Work out the finished part from the listing and answer in its coordinate system (mm). A direction names the side the tool comes from. Coordinates: 2 decimals unless noted, no trailing zeros. Order: outer loops, then holes, each group sorted by start corner. A loop starts at its lowest first (then second) coordinate and runs counter-clockwise, first axis right, second up. Notation, with made-up numbers: M 60,-7.5 L 107,-7.5 A7 cw 107,3.5 Z; hole C 60.5,68 d5. An arc over 180 degrees is marked long. Use a Markdown table: item, result.
from build123d import *

# Parameters (mm, degrees)
F0_W     = 8.736010408
F0_H     = 2.1122291218
F0_H_2   = 1.7872701865
F0_W_2   = 2.455455251
F0_H_3   = 5.8963275515
F0_W_3   = 2.8000103775
F1_DEPTH = 50
F2_DEPTH = 15
F2_TAPER = -41.9


with BuildPart() as f1:
    # F0 (on Right) → F1 (new body)
    with BuildSketch(Plane.YZ):
        with Locations((-0.0861387816, 3.9230386028)):
            Rectangle(F0_W, F0_H)
        with Locations((-0.0861387816, -3.9230386028)):
            Rectangle(F0_W, F0_H_2)
        with Locations((-5.6818716112, -0.0812397338)):
            Rectangle(F0_W_2, F0_H_3)
        with Locations((5.6818716112, -0.0812397338)):
            Rectangle(F0_W_3, F0_H_3)
        with Locations((-0.0861387816, -0.0812397338)):
            Rectangle(F0_W, F0_H_3)
    extrude(amount=F1_DEPTH)

    # F1_face (on face) → F2 (join)
    with BuildSketch(Plane(origin=(0, 0.0357904821, 0.0380455387), x_dir=(0, 1, 0), z_dir=(-1, 0, 0))):
        Polygon((-4.4899344677, -4.941107625), (4.2460759403, -4.941107625), (4.2460759403, -2.8288785031), (7.0460863178, -2.8288785031), (7.0460863178, 3.0674490483), (4.2460759403, 3.0674490483), (4.2460759403, 4.8547192348), (-4.4899344677, 4.8547192348), (-4.4899344677, 3.0674490483), (-6.9453897188, 3.0674490483), (-6.9453897188, -2.8288785031), (-4.4899344677, -2.8288785031), align=None)
    extrude(amount=F2_DEPTH, taper=F2_TAPER)


solid = f1.part
1. Flat-ended cylindrical pins translate along their axes: P1, Ø4, axis at x = 16, z = 5, coming from the -Y side; P2, Ø1.5, axis at y = -7, z = 14, coming from the +X side; P3, Ø9.5, axis at x = 23, y = 0.5, coming from the +Z side. Find the tip coordinate at first contact, or state that the pin passes through.
Answers below:
| item | result |
|---|---|
| P1 | y = -4.45 |
| P2 | x = -9.22 |
| P3 | z = 4.98 |
2. Section A-A on x = 36 is taken. Determine the outline of the cut face in (y, z).
Answers below:
| item | result |
|---|---|
| outline | M -6.91,-3.03 L -4.45,-3.03 L -4.45,-4.82 L 4.28,-4.82 L 4.28,-3.03 L 7.08,-3.03 L 7.08,2.87 L 4.28,2.87 L 4.28,4.98 L -4.45,4.98 L -4.45,2.87 L -6.91,2.87 Z |
3. For faces 1 (the face through (25, 0, -4.817)), 2 (the face through (25, -4.454, 4)), 3 (the face through (25, -6.91, 0)), 4 (the face through (25, -4.454, -4)), 5 (the face through (25, 0, 4.979)), determine the directions among +Z, -Z, +X, -X, +Y, -Y from which every point of the face is accessible in a straight line to the end or side of a thin tool.
Answers below:
| item | result |
|---|---|
| face 1 | -Z, +X, +Y, -Y |
| face 2 | +Z, +X, -Y |
| face 3 | +Z, -Z, +X, -Y |
| face 4 | -Z, +X, -Y |
| face 5 | +Z, +X, +Y, -Y |
4. Find the intervals of material crossed by probe 1 along Y at (x, z) = (33.5, -2.5); probe 2 along Z at (x, y) = (10.5, -5.5); probe 3 along Y at (x, z) = (27, 3), in increasing order.
Answers below:
| item | result |
|---|---|
| probe 1 | -6.91 to 7.08 |
| probe 2 | -3.03 to 2.87 |
| probe 3 | -4.45 to 4.28 |
